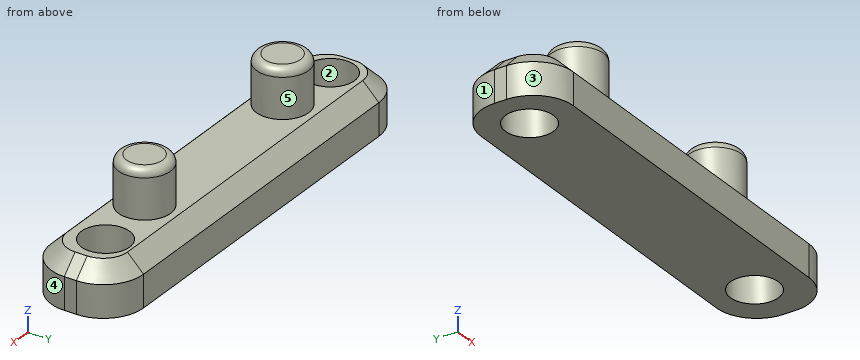
```python
from build123d import *

# Parameters (mm, degrees)
F1_DEPTH = 3
F2_R     = 1.625
F3_DEPTH = 3
F2_R_2   = 1.5
F4_DEPTH = 12.5
F5_R     = 0.5
F6_SIZE  = 1


with BuildPart() as f1:
    # F0 (on Top) → F1 (new body)
    with BuildSketch(Plane.XY):
        with BuildLine():
            Line((7.884551, 11.466584), (-13.865449, 11.466584))
            ThreePointArc((-13.865449, 11.466584), (-15.633216, 10.734351), (-16.365449, 8.966584))
            Line((-16.365449, 8.966584), (-16.365449, 8.216584))
            ThreePointArc((-16.365449, 8.216584), (-15.633216, 6.448817), (-13.865449, 5.716584))
            Line((-13.865449, 5.716584), (7.884551, 5.716584))
            ThreePointArc((7.884551, 5.716584), (9.652318, 6.448817), (10.384551, 8.216584))
            Line((10.384551, 8.216584), (10.384551, 8.966584))
            ThreePointArc((10.384551, 8.966584), (9.652318, 10.734351), (7.884551, 11.466584))
        make_face()
    extrude(amount=F1_DEPTH)

    # F2 (on face) → F3 (join)
    with BuildSketch(Plane.XY.offset(3)):
        with Locations((-9.487499, 8.421189)):
            Circle(F2_R)
        with Locations((3.262501, 8.421584)):
            Circle(F2_R)
    extrude(amount=F3_DEPTH)

    # F2 (on face) → F4 (cut, symmetric)
    with BuildSketch(Plane.XY.offset(3)):
        with Locations((-13.608467, 8.629762)):
            Circle(F2_R_2)
        with Locations((7.391072, 8.768888)):
            Circle(F2_R_2)
    extrude(amount=F4_DEPTH, both=True, mode=Mode.SUBTRACT)

    # F5
    f5_edges = [f1.edges().sort_by_distance(p)[0] for p in [
        (1.637501, 8.421584, 6),
        (-11.112499, 8.421189, 6),
    ]]
    fillet(f5_edges, radius=F5_R)

    # F6
    f6_edges = [f1.edges().sort_by_distance(p)[0] for p in [
        (-2.990449, 11.466584, 3),
        (9.652318, 10.734351, 3),
        (-15.633216, 10.734351, 3),
        (10.384551, 8.591584, 3),
        (9.652318, 6.448817, 3),
        (-2.990449, 5.716584, 3),
        (-16.365449, 8.591584, 3),
        (-15.633216, 6.448817, 3),
    ]]
    chamfer(f6_edges, length=F6_SIZE)


solid = f1.part
```
Model file for the job. Use its own axes, mm. Face numbers are marked on the shaded views. A direction names the side the tool comes from. Coordinates: 2 decimals unless noted, no trailing zeros. Loops run counter-clockwise (first coordinate to the right, second up) from the corner with the lowest first, then second, coordinate; pieces in that order, holes last. Notation, with made-up numbers: (-38.75, -28.75) - (-4.75, -28.75) arc R17 cw to (-4.75, -19.75) - close; hole circle Ø11 at (-23.5, 80.5). An arc over 180 degrees is marked (long way). Write item = value, one per line. Start each with the question number.
Item 1: Saw through at A-A, the plane z = 2.5. List the corners of the cut face in (x, y).
Item 2: Drop flat-ended pins along their axis: pin 1 Ø2.5 at (x, y) = (7.39, 8.77) entering from +Z; pin 2 Ø3 at (x, y) = (0.5, 8.5) entering from +Z. Give the stop position or say it passes through.
Item 3: Wall check: probe 1 along X at (y, z) = (9.5, 5.75); probe 2 along X at (y, z) = (9.5, 0.85); probe 3 along X at (y, z) = (8.3, 1.15). Give the ranges that are in metal, low to high. Write a range as [from, to].
Item 4: 3-axis set-ups, long thin cutter, end or side, ignore diameter. For the marked faces 4 and 5: which of +Z, -Z, +X, -X, +Y, -Y reach the whole face in a straight line?
Item 5: Pull direction Y, two halves, no side cores. Call the marked faces 1, 2 and 3: +Y half, -Y half, draft (parallel to the pull), parting line (faces both ways), or undercut.
Item 6: Saw through at B-B, the plane x = -7. List the corners of the cut face in (y, z).
Item 7: Saw through at D-D, the plane z = 0.4. List the corners of the cut face in (x, y).
Answers:
q1.outline = (-15.87, 8.22) arc R2 ccw to (-13.87, 6.22) - (7.88, 6.22) arc R2 ccw to (9.88, 8.22) - (9.88, 8.97) arc R2 ccw to (7.88, 10.97) - (-13.87, 10.97) arc R2 ccw to (-15.87, 8.97) - close; hole circle Ø3 at (-13.61, 8.63); hole circle Ø3 at (7.39, 8.77)
q2.pin_1 = through
q2.pin_2 = 5.98
q3.probe_1 = [-10.61, -8.36], [2.14, 4.39]
q3.probe_2 = [-16.31, -14.83], [-12.39, 6.08], [8.7, 10.33]
q3.probe_3 = [-16.37, -15.07], [-12.15, 5.97], [8.82, 10.38]
q4.face_4 = +Z, -Z, +X, -Y
q4.face_5 = +Z
q5.face_1 = +Y half
q5.face_2 = undercut
q5.face_3 = -Y half
q6.outline = (5.72, 0) - (11.47, 0) - (11.47, 2) - (10.47, 3) - (6.72, 3) - (5.72, 2) - close
q7.outline = (-16.37, 8.22) arc R2.5 ccw to (-13.87, 5.72) - (7.88, 5.72) arc R2.5 ccw to (10.38, 8.22) - (10.38, 8.97) arc R2.5 ccw to (7.88, 11.47) - (-13.87, 11.47) arc R2.5 ccw to (-16.37, 8.97) - close; hole circle Ø3 at (-13.61, 8.63); hole circle Ø3 at (7.39, 8.77)
